Verification items for the finished model (mm, model axes). Face numbers are marked on the shaded views. Give positions to 0.01 mm unless a question says otherwise; leave off trailing zeros. Write each loop counter-clockwise with the first axis right and the second up, starting at its lowest first coordinate (ties: lowest second). Pieces come first, ordered by that corner, then holes.
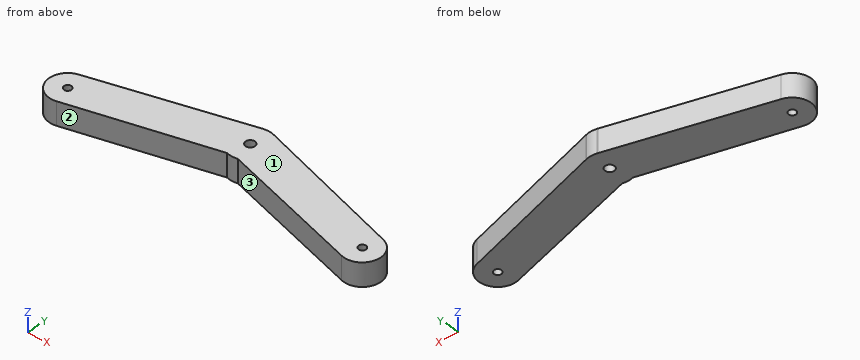
from build123d import *

# Parameters (mm, degrees)
F0_R     = 4
F0_R_2   = 5
F1_DEPTH = 25


with BuildPart() as f1:
    # F0 (on Top) → F1 (new body)
    with BuildSketch(Plane.XY):
        with BuildLine():
            Line((-6.478907, 64.423181), (-165.176381, 19.318517))
            ThreePointArc((-165.176381, 19.318517), (-179.318517, -5.176381), (-154.823619, -19.318517))
            ThreePointArc((-154.823619, -19.318517), (-154.759725, -19.301283), (-154.695889, -19.283838))
            Line((-154.695889, -19.283838), (-5.824494, 21.134565))
            ThreePointArc((-5.824494, 21.134565), (0, 20.367755), (5.824494, 21.134565))
            Line((5.824494, 21.134565), (154.695889, -19.283838))
            ThreePointArc((154.695889, -19.283838), (154.759725, -19.301283), (154.823619, -19.318517))
            ThreePointArc((154.823619, -19.318517), (179.318517, -5.176381), (165.176381, 19.318517))
            Line((165.176381, 19.318517), (6.478907, 64.423181))
            Line((6.478907, 64.423181), (5.824494, 64.609177))
            ThreePointArc((5.824494, 64.609177), (0, 65.375986), (-5.824494, 64.609177))
            Line((-5.824494, 64.609177), (-6.478907, 64.423181))
        make_face()
        with Locations((-160, 0)):
            Circle(F0_R, mode=Mode.SUBTRACT)
        with Locations((160, 0)):
            Circle(F0_R, mode=Mode.SUBTRACT)
        with Locations((0, 42.871871)):
            Circle(F0_R_2, mode=Mode.SUBTRACT)
    extrude(amount=F1_DEPTH)


solid = f1.part
Item 1: Sectioned sample at D-D on x = 113. Record the cut outline in (y, z).
Answer key:
outline: (-7.96, 0) - (34.15, 0) - (34.15, 25) - (-7.96, 25) - close
Item 2: Sectioned sample at A-A on x = 0. Record the cut outline in (y, z).
Answer key:
outline: (20.37, 0) - (37.87, 0) - (37.87, 25) - (20.37, 25) - close; (47.87, 0) - (65.38, 0) - (65.38, 25) - (47.87, 25) - close
Item 3: Sectioned sample at C-C on z = 18.5. Record the cut outline in (x, y), then the cut area to 3 significant figures.
Answer key:
outline: (-165.18, 19.32) arc R20 ccw to (-154.82, -19.32) arc R20.01 ccw to (-154.7, -19.28) - (-5.82, 21.13) arc R22.5 ccw to (5.82, 21.13) - (154.7, -19.28) arc R20.01 ccw to (154.82, -19.32) arc R20 ccw to (165.18, 19.32) - (6.48, 64.42) - (5.82, 64.61) arc R22.5 ccw to (-5.82, 64.61) - (-6.48, 64.42) - close; hole circle Ø8 at (-160, 0); hole circle Ø10 at (0, 42.87); hole circle Ø8 at (160, 0)
area: 14,700 mm2
Item 4: Release check for a two-part mould opening along X. For the marked faces 1, 2 and 3 record: released by +X, released by -X, zero draft, split by the parting line, or undercut.
Answer key:
face 1: zero draft
face 2: undercut
face 3: undercut
Item 5: Depth check by flat-ended pin: pin 1 (2 mm diameter, centred on x = -112.5, z = 11.5, fed in from -Y); pin 2 (1.5 mm diameter, centred on y = -2.5, z = 16.5, fed in from +X); pin 3 (1.5 mm diameter, centred on x = 47, z = 20, fed in from +Y). Enter the tip coordinate at first touch or a pass-through.
Answer key:
pin 1: stops at y = -8.1
pin 2: stops at x = 179.92
pin 3: stops at y = 53.12
Item 6: Sectioned sample at B-B on y = -8.5. Record the cut outline in (x, z), then the cut area to 3 significant figures.
Answer key:
outline: (-178.1, 0) - (-114.98, 0) - (-114.98, 25) - (-178.1, 25) - close; (114.98, 0) - (178.1, 0) - (178.1, 25) - (114.98, 25) - close
area: 3,160 mm2
Item 7: Scan lines: line 1 along Y through (x, z) = (-160, 19); line 2 along Y through (x, z) = (-163, 1.5); line 3 along Y through (x, z) = (138, 8.25). Record each from-to range of solid material in increasing order.
Answer key:
line 1: y = -20 to -4, 4 to 20.79
line 2: y = -19.77 to -2.65, 2.65 to 19.94
line 3: y = -14.75 to 27.04
